```python
from build123d import *

# Parameters (mm, degrees)
CROQUIS1_W                   = 30
CROQUIS1_H                   = 10
SALIENTE_EXTRUIR1_DEPTH      = 2
SALIENTE_EXTRUIR2_DEPTH      = 10
SALIENTE_EXTRUIR2_DEPTH_BACK = 2
CROQUIS2_W                   = 30
CROQUIS2_H                   = 2
CHAFL_N1_SIZE                = 2
REDONDEO2_R                  = 1
CHAFL_N2_SIZE                = 2
CORTAR_EXTRUIR1_DEPTH        = 1.2


with BuildPart() as part:
    # Croquis1 → Saliente-Extruir1 (new body)
    with BuildSketch(Plane(origin=(0, 0, 0), x_dir=(1, 0, 0), z_dir=(0, 1, 0))):
        Rectangle(CROQUIS1_W, CROQUIS1_H)
    extrude(amount=SALIENTE_EXTRUIR1_DEPTH)

    # Croquis2 → Saliente-Extruir2 (add, two sides: drawn at the far end of the back side and taken through both)
    with BuildSketch(Plane(origin=(0, 2, 0), x_dir=(1, 0, 0), z_dir=(0, 1, 0)).offset(-SALIENTE_EXTRUIR2_DEPTH_BACK)):
        with Locations((0, 6)):
            Rectangle(CROQUIS2_W, CROQUIS2_H)
    extrude(amount=SALIENTE_EXTRUIR2_DEPTH + SALIENTE_EXTRUIR2_DEPTH_BACK)

    # Chaflán1
    chafl_n1_edges = [part.edges().sort_by_distance(p)[0] for p in [
        (0, 12, -7),
    ]]
    chamfer(chafl_n1_edges, length=CHAFL_N1_SIZE - 0.0001)  # a hair under: the kernel refuses the full size

    # Redondeo2
    redondeo2_edges = [part.edges().sort_by_distance(p)[0] for p in [
        (0, 0, -7),
    ]]
    fillet(redondeo2_edges, radius=REDONDEO2_R)

    # Chaflán2
    chafl_n2_edges = [part.edges().sort_by_distance(p)[0] for p in [
        (0, 0, 5),
    ]]
    chamfer(chafl_n2_edges, length=CHAFL_N2_SIZE - 0.0001)  # a hair under: the kernel refuses the full size

    # Croquis3 → Cortar-Extruir1 (cut)
    # profile 1 of 4: a face of its own
    with BuildSketch(Plane(origin=(0, 0, -7), x_dir=(-1, 0, 0), z_dir=(0, 0, -1))):
        with BuildLine():
            ThreePointArc((2.179461585, 1.712836764), (-0.003829875, 1.526509248), (-2.187121335, 1.712836764))
            ThreePointArc((-2.187121335, 1.712836764), (-3.13057186, 3.360317888), (-3.474170032, 5.227463636))
            Line((-3.474170032, 5.227463636), (-2.805590027, 5.46631384))
            Line((-2.805590027, 5.46631384), (-2.500896715, 7.575051077))
            ThreePointArc((-2.500896715, 7.575051077), (0.006930249, 8.492471905), (2.514756719, 7.575049726))
            Line((2.514756719, 7.575049726), (2.800592253, 5.46631384))
            Line((2.800592253, 5.46631384), (3.47129645, 5.243848676))
            ThreePointArc((3.47129645, 5.243848676), (3.146201029, 3.360968701), (2.179461585, 1.712836764))
        make_face()
        with BuildLine():
            ThreePointArc((3.04052308, 4.945192572), (2.706972006, 3.446787944), (1.968364572, 2.101079281))
            ThreePointArc((1.968364572, 2.101079281), (0.001181819, 1.952323974), (-1.966000935, 2.101079281))
            ThreePointArc((-1.966000935, 2.101079281), (-2.687956628, 3.454054765), (-3.046105657, 4.945192572))
            ThreePointArc((-3.046105657, 4.945192572), (-2.637562578, 5.123424768), (-2.352779772, 5.46631384))
            Line((-2.352779772, 5.46631384), (-2.105696131, 7.381547512))
            ThreePointArc((-2.105696131, 7.381547512), (0.008132207, 8.005941127), (2.121960546, 7.381547512))
            Line((2.121960546, 7.381547512), (2.381567187, 5.46631384))
            ThreePointArc((2.381567187, 5.46631384), (2.633474347, 5.107665237), (3.04052308, 4.945192572))
        make_face(mode=Mode.SUBTRACT)
    # profile 2 of 4: a face of its own
    with BuildSketch(Plane(origin=(0, 0, -7), x_dir=(-1, 0, 0), z_dir=(0, 0, -1))):
        with BuildLine():
            Line((2.92199069, 8.735458595), (2.92199069, 6.324796966))
            ThreePointArc((2.92199069, 6.324796966), (3.056721571, 5.999527847), (3.38199069, 5.864796966))
            Line((3.38199069, 5.864796966), (3.880095869, 5.864796966))
            ThreePointArc((3.880095869, 5.864796966), (4.205364988, 5.999527847), (4.340095869, 6.324796966))
            Line((4.340095869, 6.324796966), (4.340095869, 8.735458595))
            ThreePointArc((4.340095869, 8.735458595), (4.205364988, 9.060727715), (3.880095869, 9.195458595))
            Line((3.880095869, 9.195458595), (3.38199069, 9.195458595))
            ThreePointArc((3.38199069, 9.195458595), (3.056721571, 9.060727715), (2.92199069, 8.735458595))
        make_face()
        with BuildLine():
            ThreePointArc((3.47129645, 8.849051475), (3.398492736, 8.818895189), (3.36833645, 8.746091475))
            Line((3.36833645, 8.746091475), (3.36833645, 6.314164086))
            ThreePointArc((3.36833645, 6.314164086), (3.398492736, 6.241360372), (3.47129645, 6.211204086))
            Line((3.47129645, 6.211204086), (3.923270109, 6.211204086))
            ThreePointArc((3.923270109, 6.211204086), (3.996073823, 6.241360372), (4.026230109, 6.314164086))
            Line((4.026230109, 6.314164086), (4.026230109, 8.746091475))
            ThreePointArc((4.026230109, 8.746091475), (3.996073823, 8.818895189), (3.923270109, 8.849051475))
            Line((3.923270109, 8.849051475), (3.47129645, 8.849051475))
        make_face(mode=Mode.SUBTRACT)
    # profile 3 of 4: a face of its own
    with BuildSketch(Plane(origin=(0, 0, -7), x_dir=(-1, 0, 0), z_dir=(0, 0, -1))):
        Polygon((1.255664584, 4.877844546), (0.417947415, 2.921183382), (-0.779631115, 2.921183382), (-0.18084185, 4.441551322), (-1.228472775, 4.441551322), (0.599464258, 7.052448867), (0.113938081, 4.877844546), align=None)
    # profile 4 of 4: a face of its own
    with BuildSketch(Plane(origin=(0, 0, -7), x_dir=(-1, 0, 0), z_dir=(0, 0, -1))):
        with BuildLine():
            Line((-4.462655299, 8.747249221), (-4.462655299, 6.336587592))
            ThreePointArc((-4.462655299, 6.336587592), (-4.308523171, 5.964479719), (-3.936415299, 5.810347592))
            Line((-3.936415299, 5.810347592), (-3.43831012, 5.810347592))
            ThreePointArc((-3.43831012, 5.810347592), (-3.066202247, 5.964479719), (-2.91207012, 6.336587592))
            Line((-2.91207012, 6.336587592), (-2.91207012, 8.747249221))
            ThreePointArc((-2.91207012, 8.747249221), (-3.066202247, 9.119357093), (-3.43831012, 9.273489221))
            Line((-3.43831012, 9.273489221), (-3.936415299, 9.273489221))
            ThreePointArc((-3.936415299, 9.273489221), (-4.308523171, 9.119357093), (-4.462655299, 8.747249221))
        make_face()
        with BuildLine():
            ThreePointArc((-3.939103691, 8.842918202), (-4.002743301, 8.816557812), (-4.029103691, 8.752918202))
            Line((-4.029103691, 8.752918202), (-4.029103691, 6.320990813))
            ThreePointArc((-4.029103691, 6.320990813), (-4.002743301, 6.257351203), (-3.939103691, 6.230990813))
            Line((-3.939103691, 6.230990813), (-3.544021822, 6.230990813))
            ThreePointArc((-3.544021822, 6.230990813), (-3.480382211, 6.257351203), (-3.454021822, 6.320990813))
            Line((-3.454021822, 6.320990813), (-3.454021822, 8.752918202))
            ThreePointArc((-3.454021822, 8.752918202), (-3.480382211, 8.816557812), (-3.544021822, 8.842918202))
            Line((-3.544021822, 8.842918202), (-3.939103691, 8.842918202))
        make_face(mode=Mode.SUBTRACT)
    extrude(amount=-CORTAR_EXTRUIR1_DEPTH, mode=Mode.SUBTRACT)


solid = part.part
```
For this review, take the finished solid that the model builds, in its own axes (mm). A direction names the side the tool comes from. Give positions to 0.01 mm unless a question says otherwise; leave off trailing zeros. Loops run counter-clockwise (first coordinate to the right, second up) from the corner with the lowest first, then second, coordinate; pieces in that order, holes last. Notation, with made-up numbers: M 55.25,46.25 L 96.25,46.25 A28 ccw 96.25,85.25 Z; hole C 53.5,77.25 d9. An arc over 180 degrees is marked long. One line per item, written item: value. Start each with the question number.
Q1. Machinability: for faces 4 (the face through (0, 2, 0)), 5 (the face through (2.68, 3.43, -6.41)), 6 (the face through (15, 1.5, -3.2)), which of the approach directions +Z, -Z, +X, -X, +Y, -Y give a long, thin tool a straight path to every point of the face, cutting with its end or side? Answer none if there is none.
Q2. Draft analysis for pull direction X (two halves, no side actions). For faces 1 (the face through (-4, 5, -7)), 2 (the face through (-1, 4.878, -6)), 3 (the face through (-15, 1.5, -3.2)), state which applies: released by +X, released by -X, zero draft, split by the parting line, or undercut.
Q3. Add section C-C (z = 1.25). Give the boundary of the cut face in (x, y).
Q4. Clearance check with flat-ended pins moving along their axes: pin 1 Ø6 at (x, y) = (3, 4) entering from -Z; pin 2 Ø0.5 at (x, z) = (-3.5, -6.5) entering from +Y; pin 3 Ø5 at (x, y) = (8, 5.5) entering from +Z; pin 4 Ø1.3 at (x, z) = (0, -6.5) entering from +Y. State where each tip first meets the part, or that it passes through.
Q5. For L1, parallel to X at y = 3.75, z = -6; L2, parallel to Z at x = 1.5, y = 9.25; L3, parallel to Y at x = -7.5, z = -4, list the stretches that pass through material, from the lowest coordinate up.
Q6. Add section B-B (y = 2.5). Give the boundary of the cut face in (x, z).
Q7. Add section D-D (z = 4.25). Give the boundary of the cut face in (x, y).
Reply:
1. face 4: +Z, +X, -X, +Y
1. face 5: -Z
1. face 6: +Z, -Z, +X, +Y, -Y
2. face 1: zero draft
2. face 2: undercut
2. face 3: released by -X
3. outline: M -15,0 L 15,0 L 15,2 L -15,2 Z
4. pin 1: z = -7
4. pin 2: y = 10.75
4. pin 3: z = -5
4. pin 4: y = 11.15
5. L1: -15 to -3.27, -2.81 to -0.77, 0.45 to 2.79, 3.26 to 15
5. L2: -7 to -5
5. L3: 0 to 2
6. outline: M -15,-7 L -2.74,-7 L -2.74,-5.8 L -2.24,-5.8 L -2.24,-7 L 2.23,-7 L 2.23,-5.8 L 2.73,-5.8 L 2.73,-7 L 15,-7 L 15,-5 L -15,-5 Z
7. outline: M -15,1.25 L 15,1.25 L 15,2 L -15,2 Z
